The listing builds one solid part. Answer for the finished solid, in the listing's coordinates (mm). A direction names the side the tool comes from. Give positions to 0.01 mm unless a question says otherwise; leave off trailing zeros. Write each loop counter-clockwise with the first axis right and the second up, starting at its lowest first coordinate (ties: lowest second). Pieces come first, ordered by that corner, then holes. Notation, with made-up numbers: (2.5, 54) -> (26.5, 54) arc R16 ccw to (26.5, 85) -> close; hole circle Ø8 at (41.5, 0.5). An arc over 180 degrees is marked (long way). One line per question, with ' | ' between items.
from build123d import *

# Parameters (mm, degrees)
SKETCH1_R                = 6
BOSS_EXTRUDE1_DEPTH      = 104
BOSS_EXTRUDE1_DEPTH_BACK = 36
CUT_EXTRUDE3_START       = -36
SKETCH2_W                = 4
SKETCH2_H                = 5
CUT_EXTRUDE3_DEPTH       = 20
CUT_EXTRUDE3_DEPTH_BACK  = 0.0001
CUT_EXTRUDE4_START       = 104
SKETCH2_2_W              = 4
SKETCH2_2_H              = 5
CUT_EXTRUDE4_DEPTH       = 50
CUT_EXTRUDE6_START       = -36
SKETCH3_W                = 4
SKETCH3_H                = 10
CUT_EXTRUDE6_DEPTH       = 6


with BuildPart() as part:
    # Sketch1 → Boss-Extrude1 (new body, two sides)
    with BuildSketch(Plane(origin=(0, 0, 0), x_dir=(1, 0, 0), z_dir=(0, 1, 0))) as boss_extrude1_sk:
        Circle(SKETCH1_R)
    extrude(amount=BOSS_EXTRUDE1_DEPTH)
    extrude(boss_extrude1_sk.sketch, amount=-BOSS_EXTRUDE1_DEPTH_BACK)

    # Sketch2 → Cut-Extrude3 (cut, two sides)
    with BuildSketch(Plane(origin=(0, 0, 0), x_dir=(1, 0, 0), z_dir=(0, 1, 0)).offset(CUT_EXTRUDE3_START)) as cut_extrude3_sk:
        with Locations((0, -6)):
            Rectangle(SKETCH2_W, SKETCH2_H)
    extrude(amount=CUT_EXTRUDE3_DEPTH, mode=Mode.SUBTRACT)
    extrude(cut_extrude3_sk.sketch, amount=-CUT_EXTRUDE3_DEPTH_BACK, mode=Mode.SUBTRACT)

    # Sketch2<2> → Cut-Extrude4 (cut)
    with BuildSketch(Plane(origin=(0, 0, 0), x_dir=(1, 0, 0), z_dir=(0, 1, 0)).offset(CUT_EXTRUDE4_START)):
        with Locations((0, -6)):
            Rectangle(SKETCH2_2_W, SKETCH2_2_H)
    extrude(amount=-CUT_EXTRUDE4_DEPTH, mode=Mode.SUBTRACT)

    # Sketch3 → Cut-Extrude6 (cut)
    with BuildSketch(Plane(origin=(0, 0, 0), x_dir=(1, 0, 0), z_dir=(0, 1, 0)).offset(CUT_EXTRUDE6_START)):
        with Locations((0, -6)):
            Rectangle(SKETCH3_W, SKETCH3_H)
    extrude(amount=CUT_EXTRUDE6_DEPTH, mode=Mode.SUBTRACT)


solid = part.part
Item 1: Find section C-C (y = 52). Write down the section's boundary in (x, z), then the cut area to 3 significant figures.
Answers below:
outline: circle Ø12 at (0, 0) | area: 113 mm²
Item 2: Consider line 1 (Y direction, x = -1.75, z = 1.5); line 2 (X direction, y = 10, z = -0.5); line 3 (X direction, y = 12.5, z = 1.75). Determine where each line is inside the solid, lowest interval first. Write a range as [from, to].
Answers below:
line 1: [-30, 104] | line 2: [-5.98, 5.98] | line 3: [-5.74, 5.74]
Item 3: Flat-ended cylindrical pins translate along their axes: pin 1 (1.1 mm diameter, centred on y = 81.5, z = 5, fed in from -X); pin 2 (1.2 mm diameter, centred on x = 0.5, y = -26, fed in from +Z); pin 3 (2 mm diameter, centred on y = 1, z = 3.5, fed in from -X). Find the tip coordinate at first contact, or state that the pin passes through.
Answers below:
pin 1: x = -4.02 | pin 2: z = 3.5 | pin 3: x = -5.45
Item 4: Find section B-B (z = 2.25). Write down the section's boundary in (x, y), then the cut area to 3 significant figures.
Answers below:
outline: (-5.56, -36) -> (-2, -36) -> (-2, -30) -> (2, -30) -> (2, -36) -> (5.56, -36) -> (5.56, 104) -> (-5.56, 104) -> close | area: 1,530 mm²
Item 5: Find section D-D (y = -21). Write down the section's boundary in (x, z), then the cut area to 3 significant figures.
Answers below:
outline: (-2, 3.5) -> (-2, 5.66) arc R6 ccw (long way) to (2, 5.66) -> (2, 3.5) -> close | area: 104 mm²
Item 6: Find section A-A (x = 0). Write down the section's boundary in (y, z), then the cut area to 3 significant figures.
Answers below:
outline: (-36, -6) -> (104, -6) -> (104, 3.5) -> (54, 3.5) -> (54, 6) -> (-16, 6) -> (-16, 3.5) -> (-30, 3.5) -> (-30, 1) -> (-36, 1) -> close | area: 1,490 mm²
Item 7: A tool of negligible diameter and unlimited length cuts with its end or side. For faces 1 (the face through (2, -28, 4)), 2 (the face through (0, 104, 0)), 3 (the face through (0, 79, 3.5)), from which of +Z, -Z, +X, -X, +Y, -Y can it reach the whole face along a straight path? Write none if from no direction.
Answers below:
face 1: +Z, -Y | face 2: +Z, -Z, +X, -X, +Y | face 3: +Z, +Y
Item 8: Determine the mould class of faces 4 (the face through (0, -30, 2)), 5 (the face through (0, -36, 0)), 6 (the face through (-0.78, 34.98, -5.95)), 7 (the face through (0, -33, 1)) for opening direction X: pulls with the +X half, pulls with the -X half, needs draft (parallel to the pull), parting line crosses it, or undercut.
Answers below:
face 4: undercut | face 5: needs draft | face 6: parting line crosses it | face 7: undercut
